Work out the finished part from the listing and answer in its coordinate system (mm). A direction names the side the tool comes from. Coordinates: 2 decimals unless noted, no trailing zeros. Order: outer loops, then holes, each group sorted by start corner. A loop starts at its lowest first (then second) coordinate and runs counter-clockwise, first axis right, second up. Notation, with made-up numbers: M 35.25,47 L 54.25,47 A3 ccw 54.25,52 Z; hole C -23,89 d7. An arc over 180 degrees is marked long. Use a Markdown table: item, result.
from build123d import *

# Parameters (mm, degrees)
SKETCH1_W            = 76.2
SKETCH1_H            = 76.2
BOSS_EXTRUDE1_DEPTH  = 5
FILLET1_R            = 5.334
BOSS_EXTRUDE2_DEPTH  = 5
M4_CLEARANCE_HOLE1_D = 4.8


with BuildPart() as part:
    # Sketch1 → Boss-Extrude1 (new body)
    with BuildSketch(Plane.XY):
        Rectangle(SKETCH1_W, SKETCH1_H)
    extrude(amount=BOSS_EXTRUDE1_DEPTH)

    # Fillet1
    fillet1_edges = [part.edges().sort_by_distance(p)[0] for p in [
        (38.1, -38.1, 2.5),
        (-38.1, -38.1, 2.5),
        (-38.1, 38.1, 2.5),
        (38.1, 38.1, 2.5),
    ]]
    fillet(fillet1_edges, radius=FILLET1_R)

    # Sketch2 → Boss-Extrude2 (add)
    with BuildSketch(Plane.XY.offset(5)):
        with BuildLine():
            Line((-38.1, -30.090129163), (-41.393974839, -33.620461233))
            ThreePointArc((-41.393974839, -33.620461233), (-41.250124596, -41.273219147), (-33.596647392, -41.371622715))
            Line((-33.596647392, -41.371622715), (-30.131751686, -38.1))
            Line((-30.131751686, -38.1), (-5.5, -38.1))
            Line((-5.5, -38.1), (-5.5, -41.7647))
            ThreePointArc((-5.5, -41.7647), (0, -47.2647), (5.5, -41.7647))
            Line((5.5, -41.7647), (5.5, -38.1))
            Line((5.5, -38.1), (30.131751686, -38.1))
            Line((30.131751686, -38.1), (33.596647392, -41.371622715))
            ThreePointArc((33.596647392, -41.371622715), (41.250124596, -41.273219147), (41.393974839, -33.620461233))
            Line((41.393974839, -33.620461233), (38.1, -30.090129163))
            Line((38.1, -30.090129163), (38.1, -5.5))
            Line((38.1, -5.5), (41.7647, -5.5))
            ThreePointArc((41.7647, -5.5), (47.2647, 0), (41.7647, 5.5))
            Line((41.7647, 5.5), (38.1, 5.5))
            Line((38.1, 5.5), (38.1, 30.090129163))
            Line((38.1, 30.090129163), (41.393974839, 33.620461233))
            ThreePointArc((41.393974839, 33.620461233), (41.250124596, 41.273219147), (33.596647392, 41.371622715))
            Line((33.596647392, 41.371622715), (30.131751686, 38.1))
            Line((30.131751686, 38.1), (5.5, 38.1))
            Line((5.5, 38.1), (5.5, 41.7647))
            ThreePointArc((5.5, 41.7647), (0, 47.2647), (-5.5, 41.7647))
            Line((-5.5, 41.7647), (-5.5, 38.1))
            Line((-5.5, 38.1), (-30.131751686, 38.1))
            Line((-30.131751686, 38.1), (-33.596647392, 41.371622715))
            ThreePointArc((-33.596647392, 41.371622715), (-41.250124596, 41.273219147), (-41.393974839, 33.620461233))
            Line((-41.393974839, 33.620461233), (-38.1, 30.090129163))
            Line((-38.1, 30.090129163), (-38.1, 5.5))
            Line((-38.1, 5.5), (-41.7647, 5.5))
            ThreePointArc((-41.7647, 5.5), (-47.2647, 0), (-41.7647, -5.5))
            Line((-41.7647, -5.5), (-38.1, -5.5))
            Line((-38.1, -5.5), (-38.1, -30.090129163))
        make_face()
    extrude(amount=-BOSS_EXTRUDE2_DEPTH)

    # M4 Clearance Hole1 (through all)
    with Locations(Plane.XY.offset(5)):
        with Locations((0, -41.7647), (37.372601718, -37.372601718), (-37.372601718, -37.372601718), (-41.7647, 0), (41.7647, 0), (37.372601718, 37.372601718), (0, 41.7647), (-37.372601718, 37.372601718)):
            Hole(M4_CLEARANCE_HOLE1_D / 2)


solid = part.part
(1) Straight lines are drawn through the part: L1, parallel to X at y = -37.5, z = 1.9; L2, parallel to Y at x = -0.5, z = 1.2; L3, parallel to Y at x = -40.5, z = 4.15. For each, find the intervals that lie inside material, in ascending order.
Conclusion:
| item | result |
|---|---|
| L1 | -42.87 to -39.77, -34.98 to 34.98, 39.77 to 42.87 |
| L2 | -47.24 to -44.11, -39.42 to 39.42, 44.11 to 47.24 |
| L3 | -41.9 to -32.66, -5.5 to -2.04, 2.04 to 5.5, 32.66 to 41.9 |
(2) A cutting plane is placed at A-A (x = 0). Determine the outline of the cut face in (y, z).
Conclusion:
| item | result |
|---|---|
| outline | M -47.26,0 L -44.16,0 L -44.16,5 L -47.26,5 Z; M -39.36,0 L 39.36,0 L 39.36,5 L -39.36,5 Z; M 44.16,0 L 47.26,0 L 47.26,5 L 44.16,5 Z |
(3) A cutting plane is placed at C-C (y = -17). Determine the outline of the cut face in (x, z).
Conclusion:
| item | result |
|---|---|
| outline | M -38.1,0 L 38.1,0 L 38.1,5 L -38.1,5 Z |
(4) Given P1, Ø4.5, axis at x = 37.37, y = 37.37, coming from the -Z side; P2, Ø2, axis at x = 28, z = 2.5, coming from the +Y side; P3, Ø7.5, axis at x = -37.37, y = 37.37, coming from the +Z side; P4, Ø3, axis at y = -22, z = 1.5, coming from the +X side, each flat-ended and moving along its own axis, determine where each tip first touches the part or whether it passes through.
Conclusion:
| item | result |
|---|---|
| P1 | through |
| P2 | y = 38.1 |
| P3 | z = 5 |
| P4 | x = 38.1 |
(5) Which of the six approach directions +Z, -Z, +X, -X, +Y, -Y give full straight-line access (tool end or side, diameter ignored) to faces 4 (the flat face through (-18, 38.1, 3)), 5 (the flat face through (-40, -5.5, 3)), 6 (the flat face through (38.1, -18, 3))?
Conclusion:
| item | result |
|---|---|
| face 4 | +Z, -Z, +Y |
| face 5 | +Z, -Z, -X |
| face 6 | +Z, -Z, +X |
(6) Determine the mould class of faces 1 (the cylindrical face through (0.312, 44.144, 2.465)), 2 (the flat face through (31.84, -39.713, 2.535)), 3 (the flat face through (-1, 1, 0)) for opening direction Y: pulls with the +Y half, pulls with the -Y half, needs draft (parallel to the pull), parting line crosses it, or undercut.
Conclusion:
| item | result |
|---|---|
| face 1 | undercut |
| face 2 | pulls with the -Y half |
| face 3 | needs draft |
